The model under review builds one solid part; all positions refer to its coordinate system, in mm. Face numbers are marked on the shaded views. A direction names the side the tool comes from. Give positions to 0.01 mm unless a question says otherwise; leave off trailing zeros. Loops run counter-clockwise (first coordinate to the right, second up) from the corner with the lowest first, then second, coordinate; pieces in that order, holes last. Notation, with made-up numbers: M 2.25,73 L 58.25,73 A25 cw 58.25,108 Z; hole C 66,17 d5. An arc over 180 degrees is marked long. Return JSON: item names as keys, results as strings.
Autodesk Inventor part; units mm, degrees
ref_plane "Work Plane1" through (0, 0, 10) normal (0, 0, 1) x (1, 0, 0)
ref_plane "YZ Plane" through (0, 0, 0) normal (1, 0, 0) x (0, 1, 0)
ref_plane "XZ Plane" through (0, 0, 0) normal (0, 1, 0) x (-1, 0, 0)
ref_plane "Work Plane1" through (0, 0, 10) normal (0, 0, 1) x (1, 0, 0)
sketch "Sketch1" plane through (0, 0, 10) normal (0, 0, 1) x (1, 0, 0)
  line L0 (-4.0299, -0.3538) -> (-2.2322, 1.4439) construction
  arc A0 (-1.4439, 2.2322) -> (-2.2322, 1.4439) centre (-0.9299, 0.9299) ccw construction
  line L1 (-1.4439, 2.2322) -> (0.3538, 4.0299) construction
  line L2 (-37.8299, 42.2137) -> (-37.8299, 45.8299) construction
  line L3 (-37.8299, 45.8299) -> (-4.0299, 45.8299) construction
  line L4 (-4.0299, 45.8299) -> (-4.0299, 42.2137) construction
  line L5 (-4.0299, 4.0299) -> (0.3538, 4.0299)
  circle A1 centre (-20.9299, 20.9299) radius 17.5 construction
  line L6 (-20.9299, 58.9723) -> (17.1124, 20.9299) construction
  line L7 (17.1124, 20.9299) -> (-20.9299, -17.1124) construction
  line L8 (-20.9299, -17.1124) -> (-58.9723, 20.9299) construction
  line L9 (-58.9723, 20.9299) -> (-20.9299, 58.9723) construction
  line L10 (-20.9299, 58.9723) -> (-20.9299, -17.1124) construction
  line L11 (17.1124, 20.9299) -> (-58.9723, 20.9299) construction
  line L12 (-20.9299, 58.9723) -> (32.8701, 58.9723) construction
  line L13 (-43.2198, 43.4299) -> (1.7802, 43.4299) construction
  line L14 (1.7802, 43.4299) -> (1.7802, -1.5701) construction
  line L15 (1.7802, -1.5701) -> (-43.2198, -1.5701) construction
  line L16 (-43.2198, -1.5701) -> (-43.2198, 43.4299) construction
  line L17 (-43.2198, 5.1774) -> (-43.2198, 36.6824)
  line L18 (-43.2198, 36.6824) -> (-36.4723, 43.4299)
  line L19 (-36.4723, 43.4299) -> (-5.3876, 43.4299)
  line L20 (-5.3876, 43.4299) -> (1.7802, 36.2621)
  line L21 (1.7802, 36.2621) -> (1.7802, 5.5977)
  line L22 (1.7802, 5.5977) -> (-5.3876, -1.5701)
  line L23 (-5.3876, -1.5701) -> (-36.4723, -1.5701)
  line L24 (-36.4723, -1.5701) -> (-43.2198, 5.1774)
  line L25 (-4.0299, 42.2137) -> (-37.8299, 42.2137)
  line L26 (-4.0299, -0.3538) -> (-4.0299, 4.0299)
  line L27 (-43.2198, 43.4299) -> (-10.4667, 10.6769) construction
  line L28 (-8.5595, 8.5517) -> (1.7802, -1.5701) construction
  line L29 (1.7802, 43.4299) -> (-25.699, 15.9507) construction
  line L30 (-30.9728, 10.6769) -> (-43.2198, -1.5701) construction
  point P0 (-37.8299, 4.0299)
  dimension "d18" = 53.8
  dimension "d19" = 45
  dimension "d20" = 53.8
  dimension "d21" = 45
  dimension "d22" = 45
extrude "Extrusion1" add sketch "Sketch1" along normal blind 8
sketch "Sketch3" plane through (0, 0, 10) normal (0, 0, -1) x (-1, 0, 0)
  line L0 (37.8299, -0.4701) -> (37.8299, 4.0299) construction
  line L1 (4.0299, 4.0299) -> (4.0299, -0.4701) construction
  line L2 (37.8299, -0.4701) -> (37.8299, 1.1886) construction
  line L3 (4.0299, -3.9701) -> (4.0299, -0.3538) construction
  line L4 (45.8299, 4.0299) -> (42.2137, 4.0299) construction
  line L5 (-0.3538, 4.0299) -> (-3.9701, 4.0299) construction
  line L6 (-3.9701, 37.8299) -> (-0.3538, 37.8299) construction
  line L7 (4.0299, 42.2137) -> (4.0299, 45.8299) construction
  line L8 (37.8299, 45.8299) -> (37.8299, 42.2137) construction
  line L9 (42.2137, 37.8299) -> (45.8299, 37.8299) construction
  line L10 (37.8299, 37.7299) -> (45.8299, 37.7299)
  line L11 (45.8299, 37.7299) -> (45.8299, 4.1299)
  line L12 (45.8299, 4.1299) -> (37.8299, 4.1299)
  line L13 (37.8299, 4.1299) -> (37.8299, 37.7299)
  line L14 (37.7299, 4.0299) -> (4.1299, 4.0299)
  line L15 (4.1299, 4.0299) -> (4.1299, -3.9701)
  line L16 (4.1299, -3.9701) -> (37.7299, -3.9701)
  line L17 (37.7299, -3.9701) -> (37.7299, 4.0299)
  line L18 (4.0299, 4.1299) -> (-3.9701, 4.1299)
  line L19 (-3.9701, 4.1299) -> (-3.9701, 37.7299)
  line L20 (-3.9701, 37.7299) -> (4.0299, 37.7299)
  line L21 (4.0299, 37.7299) -> (4.0299, 4.1299)
  line L22 (4.1299, 37.8299) -> (37.7299, 37.8299)
  line L23 (37.7299, 37.8299) -> (37.7299, 45.8299)
  line L24 (37.7299, 45.8299) -> (4.1299, 45.8299)
  line L25 (4.1299, 45.8299) -> (4.1299, 37.8299)
  point P0 (0, 0)
  dimension "d23" = 0.1
  dimension "d24" = 0.1
  dimension "d25" = 0.1
  dimension "d26" = 0.1
  dimension "d27" = 0.1
extrude "Extrusion3" add sketch "Sketch3" against normal up to surface (8 mm away)
sketch "Skizze12" plane through (0, 0, 10) normal (0, 0, -1) x (-1, 0, 0)
  line L0 (-0.3124, 4.1299) -> (4.1299, -0.3124)
  line L1 (4.1299, -0.3124) -> (4.1299, -3.9701)
  line L2 (4.1299, -3.9701) -> (37.7299, -3.9701) construction
  line L3 (37.7299, -3.9701) -> (37.7299, -0.3124)
  line L4 (37.7299, -0.3124) -> (42.1723, 4.1299)
  line L5 (45.8299, 4.1299) -> (42.1723, 4.1299)
  line L6 (45.8299, 37.7299) -> (45.8299, 4.1299) construction
  line L7 (42.1723, 37.7299) -> (45.8299, 37.7299)
  line L8 (42.1723, 37.7299) -> (37.7299, 42.1723)
  line L9 (37.7299, 42.1723) -> (37.7299, 45.8299)
  line L10 (37.7299, 45.8299) -> (4.1299, 45.8299) construction
  line L11 (4.1299, 45.8299) -> (4.1299, 42.1723)
  line L12 (4.1299, 42.1723) -> (-0.3124, 37.7299)
  line L13 (-3.9701, 37.7299) -> (-0.3124, 37.7299)
  line L14 (-3.9701, 4.1299) -> (-3.9701, 37.7299) construction
  line L15 (-0.3124, 4.1299) -> (-3.9701, 4.1299)
  line L16 (37.9299, -4.1701) -> (3.9299, -4.1701) construction
  line L17 (3.9299, -4.1701) -> (3.9299, -0.3953)
  line L18 (3.9299, -0.3953) -> (-0.3953, 3.9299)
  line L19 (-0.3953, 3.9299) -> (-4.1701, 3.9299)
  line L20 (-4.1701, 3.9299) -> (-4.1701, 37.9299) construction
  line L21 (-4.1701, 37.9299) -> (-0.3953, 37.9299)
  line L22 (-0.3953, 37.9299) -> (3.9299, 42.2551)
  line L23 (3.9299, 42.2551) -> (3.9299, 46.0299)
  line L24 (3.9299, 46.0299) -> (37.9299, 46.0299) construction
  line L25 (37.9299, 46.0299) -> (37.9299, 42.2551)
  line L26 (37.9299, 42.2551) -> (42.2551, 37.9299)
  line L27 (42.2551, 37.9299) -> (46.0299, 37.9299)
  line L28 (46.0299, 37.9299) -> (46.0299, 3.9299) construction
  line L29 (46.0299, 3.9299) -> (42.2551, 3.9299)
  line L30 (42.2551, 3.9299) -> (37.9299, -0.3953)
  line L31 (37.9299, -0.3953) -> (37.9299, -4.1701)
  line L32 (-3.9701, 37.7299) -> (-3.9701, 37.9299)
  line L33 (37.7299, 45.8299) -> (4.1299, 45.8299)
  line L34 (4.1299, 45.8299) -> (3.9299, 45.8299)
  line L35 (37.7299, 45.8299) -> (37.9299, 45.8299)
  line L36 (45.8299, 37.7299) -> (45.8299, 37.9299)
  line L37 (45.8299, 4.1299) -> (45.8299, 3.9299)
  line L38 (37.7299, -3.9701) -> (37.9299, -3.9701)
  line L39 (4.1299, -3.9701) -> (3.9299, -3.9701)
  line L40 (-3.9701, 4.1299) -> (-3.9701, 3.9299)
  point P0 (0, 0)
  dimension "d65" = 0.2
extrude "IM_offset" add sketch "Skizze12" against normal up to surface (8 mm away)
sketch "Sketch15" plane through (0, 0, 10) normal (0, 0, -1) x (-1, 0, 0)
  line L0 (-3.9701, 3.9299) -> (-3.9701, 37.9299)
  line L1 (-0.3953, 3.9299) -> (-3.9701, 3.9299)
  line L2 (3.9299, -0.3953) -> (-0.3953, 3.9299)
  line L3 (3.9299, -3.9701) -> (3.9299, -0.3953)
  line L4 (3.9299, -3.9701) -> (37.9299, -3.9701)
  line L5 (37.9299, -0.3953) -> (37.9299, -3.9701)
  line L6 (42.2551, 3.9299) -> (37.9299, -0.3953)
  line L7 (45.8299, 3.9299) -> (42.2551, 3.9299)
  line L8 (45.8299, 3.9299) -> (45.8299, 37.9299)
  line L9 (45.8299, 37.9299) -> (42.2551, 37.9299)
  line L10 (42.2551, 37.9299) -> (37.9299, 42.2551)
  line L11 (37.9299, 42.2551) -> (37.9299, 45.8299)
  line L12 (37.9299, 45.8299) -> (3.9299, 45.8299)
  line L13 (3.9299, 45.8299) -> (3.9299, 42.2551)
  line L14 (3.9299, 42.2551) -> (-0.3953, 37.9299)
  line L15 (-0.3953, 37.9299) -> (-3.9701, 37.9299)
  line L16 (36.1799, 36.1799) -> (5.6799, 36.1799)
  line L17 (5.6799, 36.1799) -> (5.6799, 5.6799)
  line L18 (5.6799, 5.6799) -> (36.1799, 5.6799)
  line L19 (36.1799, 5.6799) -> (36.1799, 36.1799)
  line L20 (36.1799, 36.1799) -> (5.6799, 5.6799) construction
  line L21 (5.6799, 36.1799) -> (36.1799, 5.6799) construction
  point P0 (0, 0)
  point P1 (20.9299, 20.9299)
  dimension "d73" = 30.5
  dimension "d74" = 30.5
extrude "Extrusion13" cut sketch "Sketch15" against normal blind 2 contours L19 L18 L17 L16
sketch "Sketch16" plane through (0, 0, 12) normal (0, 0, -1) x (-1, 0, 0)
  line L0 (5.6799, 36.1799) -> (36.1799, 36.1799)
  line L1 (5.6799, 5.6799) -> (5.6799, 36.1799)
  line L2 (36.1799, 5.6799) -> (5.6799, 5.6799)
  line L3 (36.1799, 36.1799) -> (36.1799, 5.6799)
  line L4 (5.6799, 5.6799) -> (5.6799, 36.1799)
  line L5 (36.1799, 36.1799) -> (36.1799, 5.6799)
  line L6 (5.6799, 5.6799) -> (36.1799, 5.6799)
  line L7 (36.1799, 5.6799) -> (36.1799, 8.6799)
  line L8 (36.1799, 8.6799) -> (5.6799, 8.6799)
  line L9 (5.6799, 8.6799) -> (5.6799, 5.6799)
  line L10 (5.6799, 36.1799) -> (36.1799, 36.1799)
  line L11 (36.1799, 36.1799) -> (5.0027, 36.1799)
  line L12 (5.0027, 36.1799) -> (5.0027, 33.1799)
  line L13 (5.0027, 33.1799) -> (36.1799, 33.1799)
  line L14 (36.1799, 33.1799) -> (36.1799, 36.1799)
  point P0 (0, 0)
  dimension "d77" = 3
  dimension "d78" = 3
extrude "Extrusion14" cut sketch "Sketch16" against normal through all contours L0 L3 L13 L1 | L1 L13 L12 L11 | L8 L3 L2 L1
sketch "Sketch17" plane through (0, 0, 12) normal (0, 0, -1) x (-1, 0, 0)
  line L0 (5.6799, 8.6799) -> (36.1799, 8.6799)
  line L1 (36.1799, 33.1799) -> (36.1799, 8.6799)
  line L2 (36.1799, 33.1799) -> (5.6799, 33.1799)
  line L3 (5.6799, 8.6799) -> (5.6799, 33.1799)
  line L4 (28.4299, 28.4299) -> (13.4299, 28.4299)
  line L5 (13.4299, 28.4299) -> (13.4299, 13.4299)
  line L6 (13.4299, 13.4299) -> (28.4299, 13.4299)
  line L7 (28.4299, 13.4299) -> (28.4299, 28.4299)
  line L8 (28.4299, 28.4299) -> (13.4299, 13.4299) construction
  line L9 (13.4299, 28.4299) -> (28.4299, 13.4299) construction
  point P0 (0, 0)
  point P1 (20.9299, 20.9299)
  dimension "d81" = 15
  dimension "d82" = 15
hole "Hole1" at (-13.4299, 13.4299, 12) at (-13.4299, 28.4299, 12) at (-28.4299, 28.4299, 12) at (-28.4299, 13.4299, 12) direction (0, 0, 1) diameter 2.8 depth 12 tip angle 118
properties part number "20_Cube_Insert_RaspiCam_v3"
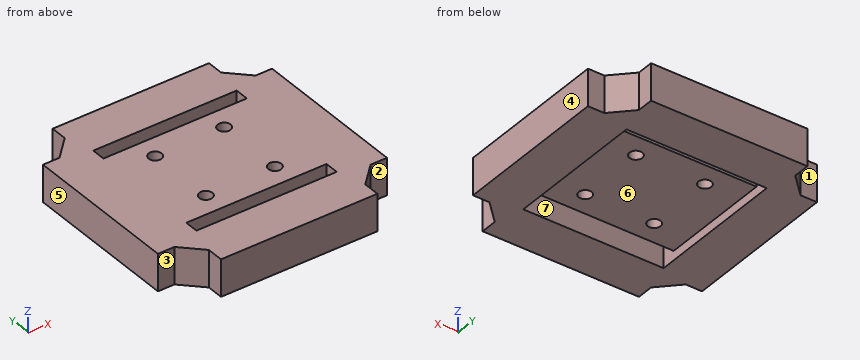
1) Wall thickness on L1, parallel to Y at x = -19.5, z = 13; L2, parallel to Y at x = -32.5, z = 11.25; L3, parallel to X at y = 33.5, z = 16.5: over which ranges is each line inside the solid? List them lowest first. Write a range as from..to.
From the geometry:
{"L1": "-3.97..5.68, 8.68..33.18, 36.18..45.83", "L2": "-3.97..5.68, 36.18..45.83", "L3": "-45.83..-36.18, -5..3.97"}
2) Consider section D-D on y = 19. Write out the cut boundary in (x, z), then the cut area to 3 significant figures.
From the geometry:
{"outline": "M -45.83,10 L -36.18,10 L -36.18,12 L -5.68,12 L -5.68,10 L 3.97,10 L 3.97,18 L -45.83,18 Z", "area": "337 mm²"}
3) Insertion check: pin 1 (12 mm diameter, centred on x = -13, y = 16, fed in from -Z); pin 2 (3 mm diameter, centred on x = -44.5, z = 15.5, fed in from -Y); pin 3 (4 mm diameter, centred on y = -2.5, z = 15.5, fed in from +X). Each pin has a flat end and moves straight along its axis. Give the tip position at first contact, or say it passes through.
From the geometry:
{"pin 1": "z = 12", "pin 2": "y = 3.93", "pin 3": "x = -3.93"}
4) Consider section A-A on x = -24. Write out the cut boundary in (y, z), then the cut area to 3 significant figures.
From the geometry:
{"outline": "M -3.97,10 L 5.68,10 L 5.68,18 L -3.97,18 Z; M 8.68,12 L 33.18,12 L 33.18,18 L 8.68,18 Z; M 36.18,10 L 45.83,10 L 45.83,18 L 36.18,18 Z", "area": "301 mm²"}
5) Tool access review of the marked faces 1, 2 and 3: name each direction out of +Z, -Z, +X, -X, +Y, -Y from which nothing blocks a thin tool from reaching the whole face with its end or side.
From the geometry:
{"face 1": "+Z, -Z, -X, +Y", "face 2": "+Z, -Z, +X, -Y", "face 3": "+Z, -Z, -X, -Y"}
6) Consider section C-C on y = 7.5. Write out the cut boundary in (x, z).
From the geometry:
{"outline": "M -45.83,10 L -36.18,10 L -36.18,18 L -45.83,18 Z; M -5.68,10 L 3.97,10 L 3.97,18 L -5.68,18 Z"}
7) Consider section B-B on z = 11. Write out the cut boundary in (x, y), then the cut area to 3 significant figures.
From the geometry:
{"outline": "M -45.83,3.93 L -42.26,3.93 L -37.93,-0.4 L -37.93,-3.97 L -3.93,-3.97 L -3.93,-0.4 L 0.4,3.93 L 3.97,3.93 L 3.97,37.93 L 0.4,37.93 L -3.93,42.26 L -3.93,45.83 L -37.93,45.83 L -37.93,42.26 L -42.26,37.93 L -45.83,37.93 Z; hole M -36.18,5.68 L -5.68,5.68 L -5.68,36.18 L -36.18,36.18 Z", "area": "1,340 mm²"}
8) The part is to be moulded in two halves that separate along X. For the marked faces 4, 5, 6 and 7, say which applies: released by +X, released by -X, zero draft, split by the parting line, or undercut.
From the geometry:
{"face 4": "released by +X", "face 5": "released by -X", "face 6": "undercut", "face 7": "undercut"}
